```python
from build123d import *

# Parameters (mm, degrees)
F1_ANGLE = 180
F2_W     = 11.076235
F2_H     = 31.188723
F3_DEPTH = 20


with BuildPart() as f1:
    # F0 (on Front) → F1 (revolve)
    with BuildSketch(Plane.XZ):
        with BuildLine():
            Line((-24.65253, 40.152624), (-9.592434, 40.152624))
            ThreePointArc((-9.592434, 40.152624), (-9.673772, 31.895267), (-7.553213, 23.914428))
            Line((-7.553213, 23.914428), (-26.719207, 23.914428))
            Line((-26.719207, 23.914428), (-26.719207, 0))
            Line((-26.719207, 0), (0, 0))
            Line((0, 0), (0, 13.119846))
            ThreePointArc((0, 13.119846), (4.151934, 9.906387), (8.790316, 7.446654))
            Line((8.790316, 7.446654), (12.329266, 19.375385))
            ThreePointArc((12.329266, 19.375385), (24.475215, 53.77601), (22.260371, 17.361432))
            Line((22.260371, 17.361432), (22.260371, 5.030416))
            ThreePointArc((22.260371, 5.030416), (33.538586, 7.754689), (43.002622, 14.466753))
            Line((43.002622, 14.466753), (71.595661, 14.466753))
            Line((71.595661, 14.466753), (71.595661, 28.638268))
            Line((71.595661, 28.638268), (50.713915, 28.638268))
            ThreePointArc((50.713915, 28.638268), (35.322294, 62.811102), (-1.652945, 56.686051))
            Line((-1.652945, 56.686051), (-24.65253, 56.686051))
            Line((-24.65253, 56.686051), (-24.65253, 40.152624))
        make_face()
    revolve(axis=Axis((-13.359603, 0, 0), (1, 0, 0)), revolution_arc=F1_ANGLE)

    # F2 (on face) → F3 (join)
    with BuildSketch(Plane(origin=(0, 0, 0), x_dir=(-1, 0, 0), z_dir=(0, 1, 0))):
        with Locations((14.0045, 1.382739)):
            Rectangle(F2_W, F2_H)
    extrude(amount=F3_DEPTH)


solid = f1.part
```
Here's how the part is built. I have some questions about the finished solid (model axes, mm). A direction names the side the tool comes from. Coordinates: 2 decimals unless noted, no trailing zeros. Order: outer loops, then holes, each group sorted by start corner. A loop starts at its lowest first (then second) coordinate and runs counter-clockwise, first axis right, second up. Notation, with made-up numbers: (7, 46.5) -> (33, 46.5) arc R23 ccw to (33, 76.5) -> close; hole circle Ø2 at (10.5, 28.5). An arc over 180 degrees is marked (long way). Return JSON: item names as keys, results as strings.
1) On a 3-axis mill with a long thin cutter (end or side, diameter ignored), from which of +Z, -Z, +X, -X, +Y, -Y can I reach the whole of each face in a straight line? I mean faces 1 (the flat face through (-8.466, 10, 1)), 2 (the conical face through (9.4, -9.5, 0.2)), 3 (the cylindrical face through (57.499, -14.463, 0.318)), 4 (the flat face through (-14, 10, 16.977)). Say none if no direction works.
Conclusion:
{"face 1": "+Z, -Z, +X, +Y", "face 2": "+Y", "face 3": "+X, +Y", "face 4": "+Z, +X, -X, +Y"}
2) Thinking about a two-plate mould opening in Y: for faces 5 (the flat face through (-26.719, -9, 0)), 6 (the cylindrical face through (-13.314, -56.672, 1.246)), 7 (the cylindrical face through (-17.27, -23.91, 0.53)), 8 (the flat face through (-14, 20, 2)), which applies, +Y half, -Y half, draft (parallel to the pull), parting line (faces both ways), or undercut?
Conclusion:
{"face 5": "draft", "face 6": "-Y half", "face 7": "undercut", "face 8": "+Y half"}
3) I'm going to push flat-ended pins straight in: P1, Ø2, axis at y = -1.5, z = -53, coming from the +X side; P2, Ø3.5, axis at x = -14, y = 7.5, coming from the +Z side; P3, Ø2, axis at y = -35, z = -3, coming from the -X side. Where does each tip first touch, or does it pass through?
Conclusion:
{"P1": "stops at x = 46.86", "P2": "stops at z = 16.98", "P3": "stops at x = -9.91"}
4) If I drill on probe 1 along Y at (x, z) = (-12.5, -19); probe 2 along Z at (x, y) = (29.5, -26); probe 3 along Y at (x, z) = (5, 56), over which ranges is the centre line in solid material (lowest first)?
Conclusion:
{"probe 1": "y = -53.41 to -35.37, -14.52 to 0", "probe 2": "z = -59.79 to -45, 45 to 59.79", "probe 3": "y = -26.77 to 0"}
5) If we section it at C-C on y = 3: List the corners of the cut face in (x, z) for me, plus the area to 3 significant figures.
Conclusion:
{"outline": "(-19.54, -14.21) -> (-8.47, -14.21) -> (-8.47, 16.98) -> (-19.54, 16.98) -> close", "area": "345 mm²"}
6) If we section it at D-D on x = 53.5: List the corners of the cut face in (y, z) for me, plus the area to 3 significant figures.
Conclusion:
{"outline": "(0, -28.64) -> (0, -14.47) arc R14.47 cw to (0, 14.47) -> (0, 28.64) arc R28.64 ccw to start", "area": "960 mm²"}
7) If we section it at B-B on z = 0: List the corners of the cut face in (x, y) for me, plus the area to 3 significant figures.
Conclusion:
{"outline": "(-26.72, -23.91) -> (-7.55, -23.91) arc R30.73 ccw to (-9.59, -40.15) -> (-24.65, -40.15) -> (-24.65, -56.69) -> (-1.65, -56.69) arc R30.73 ccw to (50.71, -28.64) -> (71.6, -28.64) -> (71.6, -14.47) -> (43, -14.47) arc R30.73 ccw to (22.26, -5.03) -> (22.26, -17.36) arc R18.42 cw (long way) to (12.33, -19.38) -> (8.79, -7.45) arc R30.73 ccw to (0, -13.12) -> (0, 0) -> (-8.47, 0) -> (-8.47, 20) -> (-19.54, 20) -> (-19.54, 0) -> (-26.72, 0) -> close", "area": "3,200 mm²"}
8) If we section it at A-A on x = 36: List the corners of the cut face in (y, z) for me, plus the area to 3 significant figures.
Conclusion:
{"outline": "(0, -62.44) -> (0, -46.15) arc R46.15 cw to (0, 46.15) -> (0, 62.44) arc R62.44 ccw to start; (0, -25.3) -> (0, -9.01) arc R9.01 cw to (0, 9.01) -> (0, 25.3) arc R25.3 ccw to start", "area": "3,660 mm²"}
